from build123d import *

# Parameters (mm, degrees)
F1_DEPTH    = 25.4
F3_T1_DEPTH = 113.1592478003
F3_T3_DEPTH = 148.0952074612


# Not quite as in the source:
# - a fillet or chamfer that OpenCascade refuses, or shapes differently, is made with other operations: its cross-section is extruded or revolved along the edge and cut away or added


with BuildPart() as f1:
    # F0 (on Right) → F1 (new body)
    with BuildSketch(Plane.YZ):
        Polygon((-103.5402726054, 0), (0, 0), (0, 6.35), (-138.112494323, 6.35), (-138.112494323, 127), (-144.462494323, 127), (-144.462494323, 0), (-109.8902726054, 0), align=None)
        Polygon((-103.5402726054, -95.25), (-103.5402726054, 0), (-109.8902726054, 0), (-109.8902726054, -101.6), (0, -101.6), (0, -95.25), align=None)
    extrude(amount=F1_DEPTH)

    # F1_face (on face) → F2 (revolve)
    with BuildSketch(Plane(origin=(25.4, -92.8938883884, -14.564984288), x_dir=(0, 1, 0), z_dir=(1, 0, 0))):
        Polygon((-51.5686059346, 14.564984288), (-16.996384217, 14.564984288), (-16.996384217, -87.035015712), (92.8938883884, -87.035015712), (92.8938883884, -80.685015712), (-10.646384217, -80.685015712), (-10.646384217, 14.564984288), (92.8938883884, 14.564984288), (92.8938883884, 20.914984288), (-45.2186059346, 20.914984288), (-45.2186059346, 141.564984288), (-51.5686059346, 141.564984288), align=None)
    revolve(axis=Axis((25.4, 0, 3.175), (0, 0, -1)))

    # F3: fillet of radius 5.08 on 4 edges, made by hand

    # F3_s2 → F3_t1 (cut)
    with BuildSketch(Plane.XY.offset(-113.1592478003)):
        with BuildLine():
            ThreePointArc((0, -106.9145079645), (1.8744370031, -109.0820354513), (4.6236991201, -109.8902726054))
            Line((4.6236991201, -109.8902726054), (4.6236991201, -109.9918726054))
            Line((4.6236991201, -109.9918726054), (0, -109.9918726054))
            Line((0, -109.9918726054), (-0.1016, -109.8902726054))
            ThreePointArc((-0.1016, -109.8902726054), (-0.1016, -108.4023902849), (-0.0924739824, -106.9565926716))
            Line((-0.0924739824, -106.9565926716), (0, -106.9145079645))
        make_face()
    extrude(amount=F3_T1_DEPTH, mode=Mode.SUBTRACT)

    # F3_s4 → F3_t3 (cut)
    with BuildSketch(Plane.XY.offset(-10.5476037306)):
        with BuildLine():
            ThreePointArc((4.2190414922, -144.462494323), (1.8281710158, -143.8646967241), (0, -142.2119976163))
            Line((0, -142.2119976163), (-0.0843808298, -142.2685876821))
            ThreePointArc((-0.0843808298, -142.2685876821), (-0.1016, -143.3372459696), (-0.1016, -144.462494323))
            Line((-0.1016, -144.462494323), (0, -144.564094323))
            Line((0, -144.564094323), (4.2190414922, -144.564094323))
            Line((4.2190414922, -144.564094323), (4.2190414922, -144.462494323))
        make_face()
    extrude(amount=F3_T3_DEPTH, mode=Mode.SUBTRACT)


solid = f1.part
Here's how the part is built. I have some questions about the finished solid (model axes, mm). A direction names the side the tool comes from. Give positions to 0.01 mm unless a question says otherwise; leave off trailing zeros. Order: outer loops, then holes, each group sorted by start corner. A loop starts at its lowest first (then second) coordinate and runs counter-clockwise, first axis right, second up. Notation, with made-up numbers: (73.5, 89.25) -> (86.5, 89.25) arc R27 cw to (86.5, 110.25) -> close; hole circle Ø9 at (12, 16). An arc over 180 degrees is marked (long way). One line per item, written item: value. Start each with the question number.
1. Imagine slicing it at D-D, the plane z = -83. List the corners of the cut face in (x, y) for me, plus the area to 3 significant figures.
2. Will these pins go through, and if not, where does the flat tip stop? pin 1 Ø23 at (x, z) = (18, -44) entering from -Y; pin 2 Ø1 at (y, z) = (31.5, 61) entering from -X; pin 3 Ø1 at (y, z) = (-77, 72.5) entering from -X.
3. For faces 4 (the face through (24, -1, 0)), 5 (the face through (100, 117, 127)), 6 (the face through (-16.085, -131.735, 67.52)), 7 (the face through (15, -109.89, -50)), which set-ups out of +Z, -Z, +X, -X, +Y, -Y let a thin tool reach every point of the face, with its end or its side?
4. We'd pull the mould along Z, two halves only. Please class faces 1 (the face through (126.478, 22.446, -46.958)), 2 (the face through (-29, -96, 0)), 3 (the face through (33.555, 109.587, -51.511)): released by +Z, released by -Z, zero draft, split by the parting line, or undercut.
5. I need wall thicknesses on probe 1 along X at (y, z) = (0, -64); probe 2 along Z at (x, y) = (65, 20); probe 3 along Y at (x, z) = (25, 93). Which ranges of each line are inside material? Lowest first, please. Write a range as from..to.
6. Imagine slicing it at C-C, the plane x = 20. List the corners of the cut face in (y, z) for me, plus the area to 3 significant figures.
7. Imagine slicing it at A-A, the plane y = 0. List the corners of the cut face in (x, z) for me.
8. Imagine slicing it at B-B, the plane z = 42.5. List the corners of the cut face in (x, y) for me, plus the area to 3 significant figures.
Values follow:
1. outline: (0, -106.91) arc R5.08 ccw to (4.62, -109.89) -> (25.4, -109.89) arc R109.89 ccw (long way) to start; hole circle Ø207.08 at (25.4, 0)
1. area: 4,280 mm2
2. pin 1: stops at y = -109.89
2. pin 2: stops at x = -115.7
2. pin 3: stops at x = -97.14
3. face 4: none
3. face 5: +Z, +X, -X, +Y, -Y
3. face 6: +Z
3. face 7: -Z, +X, -X, -Y
4. face 1: undercut
4. face 2: released by -Z
4. face 3: zero draft
5. probe 1: x = -84.49..-78.14, 128.94..135.29
5. probe 2: z = -101.6..-95.25, 0..6.35
5. probe 3: y = -144.46..-138.11, 138.11..144.46
6. outline: (-144.46, 0) -> (-109.89, 0) -> (-109.89, -101.6) -> (109.76, -101.6) -> (109.76, 0) -> (144.36, 0) -> (144.36, 127) -> (138.01, 127) -> (138.01, 6.35) -> (-138.01, 6.35) -> (-138.01, 127) -> (-144.46, 127) -> close; hole (-103.4, -95.25) -> (103.4, -95.25) -> (103.4, 0) -> (-103.4, 0) -> close
6. area: 6,000 mm2
7. outline: (-119.06, 0) -> (-84.49, 0) -> (-84.49, -101.6) -> (135.29, -101.6) -> (135.29, 0) -> (169.86, 0) -> (169.86, 127) -> (163.51, 127) -> (163.51, 6.35) -> (-112.71, 6.35) -> (-112.71, 127) -> (-119.06, 127) -> close; hole (-78.14, -95.25) -> (128.94, -95.25) -> (128.94, 0) -> (-78.14, 0) -> close
8. outline: (0, -142.21) arc R5.08 ccw to (4.22, -144.46) -> (25.4, -144.46) arc R144.46 ccw (long way) to start; hole circle Ø276.22 at (25.4, 0)
8. area: 5,650 mm2
